Geometry: final body of the model. Coordinates: model frame, mm. A direction names the side the tool comes from. Coordinates: 2 decimals unless noted, no trailing zeros. Loops run counter-clockwise (first coordinate to the right, second up) from the corner with the lowest first, then second, coordinate; pieces in that order, holes last. Notation, with made-up numbers: (50.5, -13.5) - (68.5, -13.5) arc R24 cw to (68.5, 16.5) - close; hole circle Ø8 at (-3, -21.5). An arc over 180 degrees is marked (long way). Answer in a Markdown table with one row per item.
from build123d import *

# Parameters (mm, degrees)
BOSS_EXTRUDE1_DEPTH = 2
FILLET1_R           = 2
CUT_EXTRUDE1_DEPTH  = 106.694564726
FILLET2_R           = 1
SKETCH3_W           = 2.2
SKETCH3_H           = 41
CUT_EXTRUDE2_DEPTH  = 10


with BuildPart() as part:
    # Sketch1 → Boss-Extrude1 (new body)
    with BuildSketch(Plane(origin=(0, 0, 0), x_dir=(1, 0, 0), z_dir=(0, 1, 0))):
        Polygon((0, 0), (0, 80), (10, 80), (10, 10), (60, 10), (60, 25), (70, 0), align=None)
    extrude(amount=BOSS_EXTRUDE1_DEPTH)

    # Fillet1
    fillet1_edges = [part.edges().sort_by_distance(p)[0] for p in [
        (0, 1, 0),
        (0, 1, -80),
        (10, 1, -80),
        (10, 1, -10),
        (60, 1, -10),
        (70, 1, 0),
    ]]
    fillet(fillet1_edges, radius=FILLET1_R)

    # Sketch2 → Cut-Extrude1 (cut, through all)
    with BuildSketch(Plane(origin=(0, 2, 0), x_dir=(1, 0, 0), z_dir=(0, 1, 0))):
        Polygon((60, 18.5), (62.6, 18.5), (60, 25), align=None)
    extrude(amount=-CUT_EXTRUDE1_DEPTH, mode=Mode.SUBTRACT)

    # Fillet2
    fillet2_edges = [part.edges().sort_by_distance(p)[0] for p in [
        (60, 1, -18.5),
        (62.6, 1, -18.5),
    ]]
    fillet(fillet2_edges, radius=FILLET2_R)

    # Sketch3 → Cut-Extrude2 (cut)
    with BuildSketch(Plane(origin=(0, 2, 0), x_dir=(1, 0, 0), z_dir=(0, 1, 0))):
        with Locations((5, 59.5)):
            Rectangle(SKETCH3_W, SKETCH3_H)
    extrude(amount=-CUT_EXTRUDE2_DEPTH, mode=Mode.SUBTRACT)


solid = part.part
(1) Ray query, probe 1 along X at (y, z) = (1.9, -49); probe 2 along Z at (x, y) = (35, 0.5); probe 3 along X at (y, z) = (0.1, -25). Return the intervals inside material, ascending.
Verdict:
| item | result |
|---|---|
| probe 1 | x = 0 to 3.9, 6.1 to 10 |
| probe 2 | z = -10 to 0 |
| probe 3 | x = 0 to 10 |
(2) Access query for faces 1 (the face through (60, 1, -15)), 2 (the face through (68.717, 1.014, -0.901)). Directions: +Z, -Z, +X, -X, +Y, -Y. A direction counts if a zero-diameter tool reaches every point of the face in a straight line with its end or side. Return the directions, or none.
Verdict:
| item | result |
|---|---|
| face 1 | -Z, +Y, -Y |
| face 2 | +X, +Y, -Y |
(3) Cut plane A-A on z = -62.5. Output: boundary loops of the cut face in (x, y), then the cut area to 3 significant figures.
Verdict:
| item | result |
|---|---|
| outline | (0, 0) - (3.9, 0) - (3.9, 2) - (0, 2) - close; (6.1, 0) - (10, 0) - (10, 2) - (6.1, 2) - close |
| area | 15.6 mm² |
(4) First-contact query: pin 1 Ø0.6 at (y, z) = (1, -55) entering from +X; pin 2 Ø0.5 at (x, y) = (61.5, 1) entering from -Z; pin 3 Ø1 at (x, y) = (5, 0.5) entering from -Z. Flat tips, straight axial feed; report the tip coordinate or a pass-through.
Verdict:
| item | result |
|---|---|
| pin 1 | stops at x = 10 |
| pin 2 | stops at z = -18.5 |
| pin 3 | stops at z = -39 |
(5) Cut plane D-D on x = 43.5. Output: boundary loops of the cut face in (y, z), then the cut area to 3 significant figures.
Verdict:
| item | result |
|---|---|
| outline | (0, -10) - (2, -10) - (2, 0) - (0, 0) - close |
| area | 20.0 mm² |
(6) Cut plane C-C on z = -11. Output: boundary loops of the cut face in (x, y), then the cut area to 3 significant figures.
Verdict:
| item | result |
|---|---|
| outline | (0, 0) - (10.27, 0) - (10.27, 2) - (0, 2) - close; (59.73, 0) - (65.6, 0) - (65.6, 2) - (59.73, 2) - close |
| area | 32.3 mm² |
(7) Cut plane B-B on y = 0.3. Output: boundary loops of the cut face in (x, z).
Verdict:
| item | result |
|---|---|
| outline | (0, -78) arc R2 ccw to (2, -80) - (3.9, -80) - (3.9, -39) - (6.1, -39) - (6.1, -80) - (8, -80) arc R2 ccw to (10, -78) - (10, -12) arc R2 cw to (12, -10) - (58, -10) arc R2 cw to (60, -12) - (60, -17.5) arc R1 ccw to (61, -18.5) - (61.92, -18.5) arc R1 ccw to (62.85, -17.87) - (68.9, -2.74) arc R2 ccw to (67.05, 0) - (2, 0) arc R2 ccw to (0, -2) - close |
(8) Pull-direction query (X, two-part tool) for faces 3 (the face through (6.1, 1, -59)), 4 (the face through (0.57, 1.01, -0.6)), 5 (the face through (35, 1, 0)); classes: pulls with the +X half, pulls with the -X half, needs draft (parallel to the pull), parting line crosses it, or undercut.
Verdict:
| item | result |
|---|---|
| face 3 | undercut |
| face 4 | pulls with the -X half |
| face 5 | needs draft |
